Input: dimensioned drawing with shaded views. Units: mm. Origin: part minimum x, y, z. Round coordinates to 2 decimals unless told otherwise and drop trailing zeros. Write each loop counter-clockwise with the first axis right and the second up, starting at its lowest first coordinate (ties: lowest second). Pieces come first, ordered by that corner, then holes. Notation, with made-up numbers: (12, 10) - (24, 10) arc R17 cw to (24, 22) - close; hole circle Ø6 at (-34.5, 12.5). An arc over 180 degrees is marked (long way). Use one line per item in the form item = value.
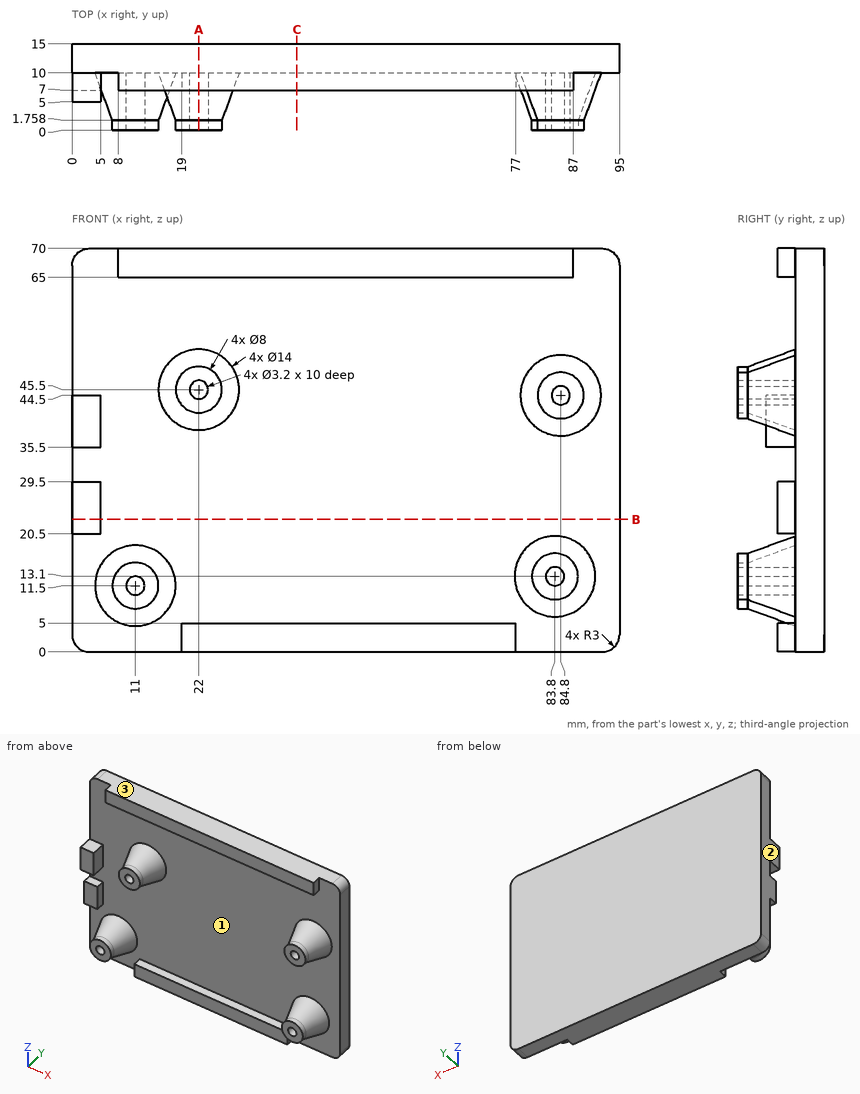
(1) Cut plane C-C on x = 39. Output: boundary loops of the cut face in (y, z), then the cut area to 3 significant figures.
Derived:
outline = (7, 0) - (15, 0) - (15, 70) - (7, 70) - (7, 65) - (10, 65) - (10, 5) - (7, 5) - close
area = 380 mm^2
(2) First-contact query: pin 1 Ø2.5 at (y, z) = (6.5, 38.5) entering from +X; pin 2 Ø3 at (x, z) = (11, 11.5) entering from -Y; pin 3 Ø1.5 at (y, z) = (7, 44.5) entering from +X; pin 4 Ø2 at (y, z) = (2, 52.5) entering from +X. Flat tips, straight axial feed; report the tip coordinate or a pass-through.
Derived:
pin_1 = 88.17
pin_2 = 10
pin_3 = 90.98
pin_4 = through
(3) Cut plane B-B on z = 23. Output: boundary loops of the cut face in (x, y).
Derived:
outline = (0, 7) - (5, 7) - (5, 10) - (95, 10) - (95, 15) - (0, 15) - close
(4) Cut plane A-A on x = 22. Output: boundary loops of the cut face in (y, z).
Derived:
outline = (0, 41.5) - (1.76, 41.5) - (10, 38.5) - (10, 5) - (7, 5) - (7, 0) - (15, 0) - (15, 70) - (7, 70) - (7, 65) - (10, 65) - (10, 52.5) - (1.76, 49.5) - (0, 49.5) - (0, 47.1) - (10, 47.1) - (10, 43.9) - (0, 43.9) - close
(5) Draft query along Z for the marked faces 1, 2 and 3. Return one class per face: released by +Z, released by -Z, zero draft, split by the parting line, or undercut.
Derived:
face_1 = undercut
face_2 = zero draft
face_3 = released by +Z
(6) Material intervals for L1, parallel to Z at x = 49, y = 8.75; L2, parallel to X at y = 9.5, z = 65.5; L3, parallel to Y at x = 11.5, z = 57.5, sorted ascending.
Derived:
L1 = 0 to 5, 65 to 70
L2 = 8 to 87
L3 = 10 to 15
